```python
from build123d import *

# Parameters (mm, degrees)
SKETCH1_R           = 6
BOSS_EXTRUDE1_DEPTH = 51.1
CHAMFER1_SIZE       = 1


with BuildPart() as part:
    # Sketch1 → Boss-Extrude1 (new body)
    with BuildSketch(Plane.XY):
        Circle(SKETCH1_R)
    extrude(amount=BOSS_EXTRUDE1_DEPTH)

    # Chamfer1
    chamfer1_edges = [part.edges().sort_by_distance(p)[0] for p in [
        (-6, 0, 0),
        (-6, 0, 51.1),
    ]]
    chamfer(chamfer1_edges, length=CHAMFER1_SIZE)

    # Groove Sketch → Retaining Ring Groove (revolve, cut)
    with BuildSketch(Plane(origin=(11.571093486, 1.818413045, 30.848914431), x_dir=(-0.1670407778174849, -0.02625068493329621, 0.9856004667646331), z_dir=(0.1552460285814813, -0.987875837648476, 0)), mode=Mode.PRIVATE) as retaining_ring_groove_sk:
        with BuildLine():
            Line((20.516209746, 14.310059643), (20.539882467, 14.448043709))
            Line((20.539882467, 14.448043709), (19.455721954, 14.634043658))
            Line((19.455721954, 14.634043658), (19.432049233, 14.496059593))
            ThreePointArc((19.432049233, 14.496059593), (19.450651377, 14.413950055), (19.521865289, 14.369043546))
            Line((19.521865289, 14.369043546), (20.3891937, 14.220243587))
            ThreePointArc((20.3891937, 14.220243587), (20.471303237, 14.238845731), (20.516209746, 14.310059643))
        make_face()
    revolve(retaining_ring_groove_sk.sketch.rotate(Axis((0, 0, 39.317134261), (0, 0, -1)), 98.931065378), axis=Axis((0, 0, 39.317134261), (0, 0, -1)), mode=Mode.SUBTRACT)

    # Groove Sketch1 → Retaining Ring Groove1 (revolve, cut)
    with BuildSketch(Plane(origin=(11.571093486, 1.818413045, 30.848914431), x_dir=(-0.16704077781748494, -0.02625068493329602, 0.9856004667646331), z_dir=(0.1552460285814813, -0.987875837648476, 0)), mode=Mode.PRIVATE) as retaining_ring_groove1_sk:
        with BuildLine():
            Line((-23.934371305, 21.93605756), (-23.910698584, 22.074041625))
            Line((-23.910698584, 22.074041625), (-24.994859097, 22.260041574))
            Line((-24.994859097, 22.260041574), (-25.018531818, 22.122057509))
            ThreePointArc((-25.018531818, 22.122057509), (-24.999929675, 22.039947971), (-24.928715762, 21.995041463))
            Line((-24.928715762, 21.995041463), (-24.061387351, 21.846241503))
            ThreePointArc((-24.061387351, 21.846241503), (-23.979277814, 21.864843647), (-23.934371305, 21.93605756))
        make_face()
    revolve(retaining_ring_groove1_sk.sketch.rotate(Axis((0, 0, 39.317134261), (0, 0, -1)), 8.931065378), axis=Axis((0, 0, 39.317134261), (0, 0, -1)), mode=Mode.SUBTRACT)


solid = part.part
```
Source: CAD feature listing. Evaluate the final solid. Frame: model axes, mm. A direction names the side the tool comes from. Coordinates: 2 decimals unless noted, no trailing zeros. Loops run counter-clockwise (first coordinate to the right, second up) from the corner with the lowest first, then second, coordinate; pieces in that order, holes last. Notation, with made-up numbers: M 72.5,-29 L 77.5,-29 A21 cw 77.5,-20 Z; hole C 79,62 d9. An arc over 180 degrees is marked long. Use CSV: the item, a comma, the result in double quotes.
(1) Contact query for flat-ended pins moving along their axis: pin 1 (4 mm diameter, centred on y = 4.5, z = 28, fed in from -X); pin 2 (1.5 mm diameter, centred on x = 2.5, z = 9.5, fed in from +Y). Output: stop coordinate, or through.
Answers follow:
pin 1,"x = -5.45"
pin 2,"y = 5.74"
(2) Draft query along Z for faces 3 (the face through (5.723, 1.802, 1.715)), 4 (the face through (0, 0, 51.1)), 5 (the face through (4.56, -3.5, 3.01)). Return one class per face: pulls with the +Z half, pulls with the -Z half, needs draft (parallel to the pull), parting line crosses it, or undercut.
Answers follow:
face 3,"needs draft"
face 4,"pulls with the +Z half"
face 5,"undercut"
(3) Cut plane A-A on z = 26. Return loops of the section in (x, y), and give its area (3 significant figures).
Answers follow:
outline,"C 0,0 d12"
area,"113 mm²"
(4) Reachability of faces 1 (the face through (5.54, -2.3, 49.36)), 2 (the face through (-5.613, -1.246, 48.106)) from +Z, -Z, +X, -X, +Y, -Y: full face, straight path, thin tool, end or side. Return the list, or none.
Answers follow:
face 1,"+Z, -Z"
face 2,"none"
(5) Line query: line 1 (Z direction, x = 5.5, y = 2); line 2 (X direction, y = -1.25, z = 41). Output: solid intervals per line, ascending. Write a range as [from, to].
Answers follow:
line 1,"[0.85, 2.45], [3.55, 47.55], [48.65, 50.25]"
line 2,"[-5.87, 5.87]"
